```python
from build123d import *

# Parameters (mm, degrees)
SKETCH_1_W          = 220
SKETCH_1_H          = 220
EXTRUDE_1_DEPTH     = 12
SKETCH_2_R          = 4.5
SKETCH_2_R_2        = 3.25
CUT_EXTRUDE_1_DEPTH = 13
SKETCH_3_R          = 5.5
CUT_EXTRUDE_2_DEPTH = 6.5


with BuildPart() as part:
    # 草图1 → 凸台-拉伸1 (new body)
    with BuildSketch(Plane.XY):
        Rectangle(SKETCH_1_W, SKETCH_1_H)
    extrude(amount=EXTRUDE_1_DEPTH)

    # 草图2 → 切除-拉伸1 (cut)
    with BuildSketch(Plane(origin=(0, 0, 0), x_dir=(-1, 0, 0), z_dir=(0, 0, -1))):
        with Locations((90, -90)):
            Circle(SKETCH_2_R)
        with Locations((90, 90)):
            Circle(SKETCH_2_R)
        with Locations((-90, -90)):
            Circle(SKETCH_2_R)
        with Locations((-90, 90)):
            Circle(SKETCH_2_R)
        with Locations((75, -75)):
            Circle(SKETCH_2_R_2)
        with Locations((75, 75)):
            Circle(SKETCH_2_R_2)
        with Locations((-75, -75)):
            Circle(SKETCH_2_R_2)
        with Locations((-75, 75)):
            Circle(SKETCH_2_R_2)
    extrude(amount=-CUT_EXTRUDE_1_DEPTH, mode=Mode.SUBTRACT)

    # 草图3 → 切除-拉伸2 (cut)
    with BuildSketch(Plane(origin=(0, 0, 0), x_dir=(-1, 0, 0), z_dir=(0, 0, -1))):
        with Locations((75, -75)):
            Circle(SKETCH_3_R)
        with Locations((75, 75)):
            Circle(SKETCH_3_R)
        with Locations((-75, -75)):
            Circle(SKETCH_3_R)
        with Locations((-75, 75)):
            Circle(SKETCH_3_R)
    extrude(amount=-CUT_EXTRUDE_2_DEPTH, mode=Mode.SUBTRACT)


solid = part.part
```
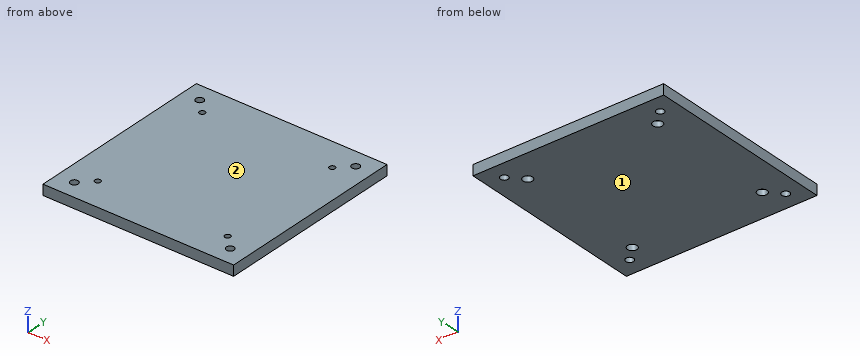
Verification items for the finished model (mm, model axes). Face numbers are marked on the shaded views. Coordinates: 2 decimals unless noted, no trailing zeros. Loops run counter-clockwise (first coordinate to the right, second up) from the corner with the lowest first, then second, coordinate; pieces in that order, holes last. Notation, with made-up numbers: (19.5, 75) - (49.5, 75) arc R8 ccw to (49.5, 82) - close; hole circle Ø3 at (34.25, 85). An arc over 180 degrees is marked (long way). Put each result on its own line as item: value.
Item 1: Gauge pin test, flat end, axial feed: pin 1 Ø3.5 at (x, y) = (73, 74.5) entering from -Z. Record the tip position at first contact, or that the pin passes through.
Conclusion:
pin 1: stops at z = 6.5
Item 2: Scan lines: line 1 along Y through (x, z) = (75, 3.25); line 2 along X through (y, z) = (90.5, 7); line 3 along Y through (x, z) = (-80, 4.75). Record each from-to range of solid material in increasing order.
Conclusion:
line 1: y = -110 to -80.5, -69.5 to 69.5, 80.5 to 110
line 2: x = -110 to -94.47, -85.53 to 85.53, 94.47 to 110
line 3: y = -110 to -77.29, -72.71 to 72.71, 77.29 to 110
Item 3: Section check A-A (x = 75). Enter the section's corners in (y, z), then the cut area to 3 significant figures.
Conclusion:
outline: (-110, 0) - (-80.5, 0) - (-80.5, 6.5) - (-78.25, 6.5) - (-78.25, 12) - (-110, 12) - close; (-71.75, 6.5) - (-69.5, 6.5) - (-69.5, 0) - (69.5, 0) - (69.5, 6.5) - (71.75, 6.5) - (71.75, 12) - (-71.75, 12) - close; (78.25, 6.5) - (80.5, 6.5) - (80.5, 0) - (110, 0) - (110, 12) - (78.25, 12) - close
area: 2,430 mm2
Item 4: Draft check along Z on the marked faces 1 and 2. Enter one of: pulls with the +Z half, pulls with the -Z half, needs draft (parallel to the pull), parting line crosses it, or undercut.
Conclusion:
face 1: pulls with the -Z half
face 2: pulls with the +Z half
